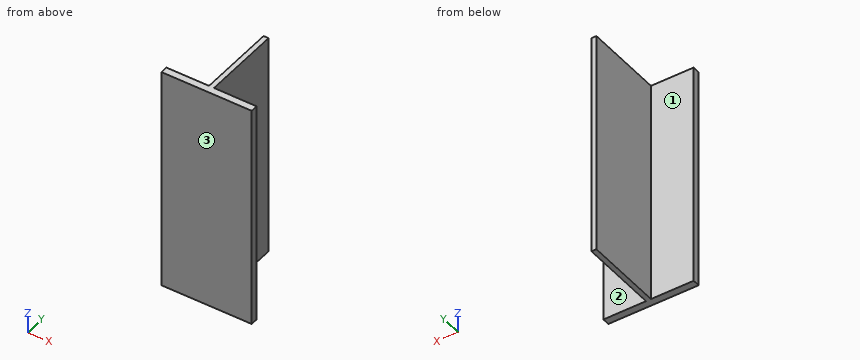
Autodesk Inventor part; units mm, degrees
ref_plane "YZ Plane" through (0, 0, 0) normal (1, 0, 0) x (0, 1, 0)
ref_plane "XZ Plane" through (0, 0, 0) normal (0, 1, 0) x (-1, 0, 0)
ref_plane "XY Plane" through (0, 0, 0) normal (0, 0, 1) x (1, 0, 0)
sketch "草圖1" plane through (0, 0, 0) normal (0, 0, 1) x (1, 0, 0)
  circle A0 centre (0, 0) radius 109.55
  line L0 (-94.8731, -54.775) -> (-98.1293, -56.655)
  line L1 (94.8731, -54.775) -> (98.1293, -56.655)
  line L2 (-117.81, 0) -> (117.81, 0)
  arc A1 (-98.1293, -56.655) -> (98.1293, -56.655) centre (0, 0) ccw
  circle A2 centre (0, 0) radius 105.79
  dimension "d0" = 219.1
  dimension "d4" = 120
  dimension "d5" = 30
  dimension "d6" = 30
  dimension "d7" = 3.76
  dimension "d12" = 3.76
sketch "草圖2" plane through (0, 0, 0) normal (0, 0, 1) x (1, 0, 0)
  line L0 (-44.45, 0) -> (44.45, 0) construction
  line L1 (-50, -209.55) -> (50, -209.55)
  line L2 (0, -109.55) -> (-51.4901, -109.55) construction
  line L3 (0, -113.31) -> (0, -136.45) construction
  line L4 (-50, -201.55) -> (-50, -209.55)
  line L5 (50, -209.55) -> (50, -201.55)
  line L6 (-50, -201.55) -> (-2.75, -201.55)
  line L7 (2.75, -201.55) -> (50, -201.55)
  line L8 (-51.4901, -113.31) -> (60.072, -113.31)
  line L9 (-2.75, -201.55) -> (-2.75, -113.31)
  line L10 (2.75, -201.55) -> (2.75, -113.31)
  arc A0 (-98.1293, -56.655) -> (98.1293, -56.655) centre (0, 0) ccw
  circle A1 centre (0, 0) radius 109.55
  point P0 (2.75, -209.55)
  point P1 (-2.75, -209.55)
  point P2 (2.75, -87.55)
  point P3 (-2.75, -87.55)
  dimension "d14" = 100
  dimension "d15" = 100
  dimension "d18" = 8
  dimension "d19" = 5.5
  dimension "d20" = 5.5
  dimension "d21" = 8
  dimension "d22" = 100
extrude "擠出3" add sketch "草圖2" along normal mid plane 250 contours L4 L6 L9 L8 L10 L7 L5 L1
equation "\"d12\" = d7"
equation "\"d14\" = Hops"
equation "\"d15\" = Section_buttom_A"
equation "\"d18\" = Section_Top_thick"
equation "\"d19\" = Section_mid_thick"
equation "\"d20\" = Section_mid_thick"
equation "\"d21\" = d18"
equation "\"d22\" = d15"
equation "\"d23\" = Lops"
equation "\"Section_buttom_A\" = 100"
equation "\"Extra_Plate_B\" = 0"
equation "\"Section_mid_thick\" = 5.5"
equation "\"Section_Top_thick\" = 8"
equation "\"Section_front_gap\" = 35"
equation "\"Section_side_Gap\" = 25"
equation "\"Hops\" = 100"
equation "\"d17\" = Section_Top_thick"
equation "\"Lops\" = Extra_Lops"
properties part number "A"
The model under review builds one solid part; all positions refer to its coordinate system, in mm. Face numbers are marked on the shaded views. A direction names the side the tool comes from. Coordinates: 2 decimals unless noted, no trailing zeros. Order: outer loops, then holes, each group sorted by start corner. A loop starts at its lowest first (then second) coordinate and runs counter-clockwise, first axis right, second up. Notation, with made-up numbers: (65.5, 11.25) -> (97.5, 11.25) arc R28 ccw to (97.5, 31.25) -> close; hole circle Ø6 at (65, -36.75). An arc over 180 degrees is marked (long way). Answer in a Markdown table with one row per item. Add a question column.
Item 1: We need section A-A on z = 9.5. Write out the cut boundary in (x, y).
Item 2: Clearance check with flat-ended pins moving along their axes: pin 1 (3 mm diameter, centred on x = 23.5, z = 37, fed in from +Y); pin 2 (6 mm diameter, centred on y = -167, z = -94.5, fed in from -X); pin 3 (3 mm diameter, centred on y = -161, z = 77, fed in from +X). State where each tip first meets the part, or that it passes through.
Item 3: Machinability: for the marked faces 1, 2 and 3, which of the approach directions +Z, -Z, +X, -X, +Y, -Y give a long, thin tool a straight path to every point of the face, cutting with its end or side? Answer none if there is none.
Item 4: We need section C-C on x = 14.5. Write out the cut boundary in (y, z).
Item 5: We need section B-B on y = -199. Write out the cut boundary in (x, z).
Item 6: To check wall thickness, follow probe 1 along X at (y, z) = (-178.5, -109.5); probe 2 along Y at (x, z) = (30.5, -84). State the ranges of each line that lie inside material, in increasing order.
Final values:
| question | item | result |
|---|---|---|
| 1 | outline | (-50, -209.55) -> (50, -209.55) -> (50, -201.55) -> (2.75, -201.55) -> (2.75, -113.31) -> (-2.75, -113.31) -> (-2.75, -201.55) -> (-50, -201.55) -> close |
| 2 | pin 1 | stops at y = -201.55 |
| 2 | pin 2 | stops at x = -2.75 |
| 2 | pin 3 | stops at x = 2.75 |
| 3 | face 1 | +Z, -Z, -X, +Y |
| 3 | face 2 | +Z, -Z, +X, +Y |
| 3 | face 3 | +Z, -Z, +X, -X, -Y |
| 4 | outline | (-209.55, -125) -> (-201.55, -125) -> (-201.55, 125) -> (-209.55, 125) -> close |
| 5 | outline | (-2.75, -125) -> (2.75, -125) -> (2.75, 125) -> (-2.75, 125) -> close |
| 6 | probe 1 | x = -2.75 to 2.75 |
| 6 | probe 2 | y = -209.55 to -201.55 |
